Verification items for the finished model (mm, model axes). Coordinates: 2 decimals unless noted, no trailing zeros. Loops run counter-clockwise (first coordinate to the right, second up) from the corner with the lowest first, then second, coordinate; pieces in that order, holes last.
Q1. Mould release check, pull along Z, two halves, no side actions. Record for faces 1 (the face through (1, -1.25, 1)), 2 (the face through (1.43, 1.102, -2.463)), 3 (the face through (-1.22, -0.02, 0.27)), 4 (the face through (1.42, 1.1, 2.47)): +Z half, -Z half, draft (parallel to the pull), parting line (faces both ways), or undercut.
Q2. Sectioned sample at B-B (y = -1.05). Enter the section's corners in (x, z).
Q3. Go/stop test with flat-tipped pins: P1, Ø1.5, axis at x = 0, z = 0, coming from the -Y side; P2, Ø1.5, axis at y = 0.5, z = -2, coming from the -X side. Record where each tip stops, or that it passes through.
Q4. Material ranges on probe 1 along X at (y, z) = (1, -0.05); probe 2 along X at (y, z) = (-0.7, -0.95); probe 3 along Z at (x, y) = (0.25, 0.1), recorded low to high.
Q5. Sectioned sample at A-A (y = 0.75). Enter the section's corners in (x, z), then the cut area to 3 significant figures.
```python
from build123d import *

# Parameters (mm, degrees)
BOSS_EXTRUDE1_DEPTH = 1.25
M3_TAPPED_HOLE1_D   = 2.5
SKETCH4_OUTSIDE_W   = 14.96
SKETCH4_OUTSIDE_H   = 14.124
SKETCH4_OUTSIDE_R   = 2.7
CUT_EXTRUDE1_DEPTH  = 2.5
CUT_EXTRUDE1_TAPER  = 45


with BuildPart() as part:
    # Sketch2 → Boss-Extrude1 (new body, symmetric)
    with BuildSketch(Plane(origin=(0, 0, 0), x_dir=(1, 0, 0), z_dir=(0, 1, 0))):
        Polygon((3.117691454, 0), (1.558845727, 2.7), (-1.558845727, 2.7), (-3.117691454, 0), (-1.558845727, -2.7), (1.558845727, -2.7), align=None)
    extrude(amount=BOSS_EXTRUDE1_DEPTH, both=True)

    # M3 Tapped Hole1 (through all)
    with Locations(Plane.ZX.offset(1.25)):
        with Locations((0, 0)):
            Hole(M3_TAPPED_HOLE1_D / 2)

    # Sketch4 outside → Cut-Extrude1 (cut)
    with BuildSketch(Plane.XZ.offset(1.25)):
        Rectangle(SKETCH4_OUTSIDE_W, SKETCH4_OUTSIDE_H)
        Circle(SKETCH4_OUTSIDE_R, mode=Mode.SUBTRACT)
    cut_extrude1 = extrude(amount=-CUT_EXTRUDE1_DEPTH, taper=CUT_EXTRUDE1_TAPER, mode=Mode.SUBTRACT)

    # Mirror1: Cut-Extrude1 across plane
    add(cut_extrude1.mirror(Plane.ZX), mode=Mode.SUBTRACT)


solid = part.part
```
Geometry check:
1. face 1: draft
1. face 2: -Z half
1. face 3: undercut
1. face 4: +Z half
2. outline: (-2.87, -0.43) - (-1.81, -2.27) arc R2.9 ccw to (-1.06, -2.7) - (1.06, -2.7) arc R2.9 ccw to (1.81, -2.27) - (2.87, -0.43) arc R2.9 ccw to (2.87, 0.43) - (1.81, 2.27) arc R2.9 ccw to (1.06, 2.7) - (-1.06, 2.7) arc R2.9 ccw to (-1.81, 2.27) - (-2.87, 0.43) arc R2.9 ccw to start; hole circle Ø2.5 at (0, 0)
3. P1: passes through
3. P2: stops at x = -2.4
4. probe 1: x = -2.95 to -1.25, 1.25 to 2.95
4. probe 2: x = -2.57 to -0.81, 0.81 to 2.57
4. probe 3: z = -2.7 to -1.22, 1.22 to 2.7
5. outline: (-3.12, 0) - (-1.56, -2.7) - (1.56, -2.7) - (3.12, 0) - (1.56, 2.7) - (-1.56, 2.7) - close; hole circle Ø2.5 at (0, 0)
5. area: 20.3 mm2
